Read the model definition and answer for the solid it produces. Units are mm, in the model's axes. A direction names the side the tool comes from. Give positions to 0.01 mm unless a question says otherwise; leave off trailing zeros. Loops run counter-clockwise (first coordinate to the right, second up) from the corner with the lowest first, then second, coordinate; pieces in that order, holes last. Notation, with made-up numbers: (-5.5, -26) -> (41.5, -26) arc R15 cw to (41.5, -2) -> close; hole circle Ø10 at (25, -38). An arc over 180 degrees is marked (long way). Return JSON: item names as keys, results as strings. Group by question number.
from build123d import *

# Parameters (mm, degrees)
F0_R     = 25.4
F1_DEPTH = 1.27
F3_R     = 1.27
F4_DEPTH = 76.2
F5_R     = 28.9937476924
F6_DEPTH = 38.1


# Not quite as in the source:
# - a fillet or chamfer that OpenCascade refuses, or shapes differently, is made with other operations: its cross-section is extruded or revolved along the edge and cut away or added


with BuildPart() as f1:
    # F0 (on Top) → F1 (new body)
    with BuildSketch(Plane.XY):
        Circle(F0_R)
    extrude(amount=F1_DEPTH)

    # F2: fillet of radius 5.08 on 1 edges, made by hand

    # F2_s1 → F2_t2 (revolve, cut)
    with BuildSketch(Plane.XZ):
        with BuildLine():
            ThreePointArc((25.4, 0), (23.8359470592, 0.9419048812), (22.0398958349, 1.27))
            Line((22.0398958349, 1.27), (25.4, 1.27))
            Line((25.4, 1.27), (25.4, 0))
        make_face()
    revolve(axis=Axis((0, 0, 1.27), (0, 0, 1)), mode=Mode.SUBTRACT)

    # F3 (on face) → F4 (join)
    with BuildSketch(Plane.XY.offset(1.27)):
        Circle(F3_R)
    extrude(amount=F4_DEPTH)

    # F5 (on face) → F6 (join)
    with BuildSketch(Plane.XY.offset(77.47)):
        with Locations((-1.27, 0)):
            Circle(F5_R)
    extrude(amount=F6_DEPTH)


solid = f1.part
1. Section B-B on x = 0 is taken. Determine the outline of the cut face in (y, z).
2. Flat-ended cylindrical pins translate along their axes: pin 1 Ø3 at (y, z) = (21.5, 85) entering from +X; pin 2 Ø4 at (y, z) = (-2.5, 90.5) entering from -X. Find the tip coordinate at first contact, or state that the pin passes through.
3. Straight lines are drawn through the part: line 1 (Z direction, x = -12.5, y = 18.5); line 2 (Z direction, x = -26, y = -2.5); line 3 (Z direction, x = 24, y = 0). For each, find the intervals that lie inside material, in ascending order. Write a range as from..to.
4. Which of the six approach directions +Z, -Z, +X, -X, +Y, -Y give full straight-line access (tool end or side, diameter ignored) to faces 1 (the cylindrical face through (-0.17, 1.26, 38.84)), 2 (the cylindrical face through (-7.555, -28.304, 96.253))?
5. Determine the mould class of faces 3 (the flat face through (-2, 0, 115.57)), 4 (the flat face through (0, 0, 0)), 5 (the flat face through (-2, 0, 77.47)) for opening direction Z: pulls with the +Z half, pulls with the -Z half, needs draft (parallel to the pull), parting line crosses it, or undercut.
6. Section A-A on z = 17.5 is taken. Determine the outline of the cut face in (x, y), then the cut area to 3 significant figures.
Completed:
{
 "1": {"outline": "(-28.97, 77.47) -> (-1.27, 77.47) -> (-1.27, 1.27) -> (-22.04, 1.27) arc R5.08 ccw to (-25.4, 0) -> (25.4, 0) arc R5.08 ccw to (22.04, 1.27) -> (1.27, 1.27) -> (1.27, 77.47) -> (28.97, 77.47) -> (28.97, 115.57) -> (-28.97, 115.57) -> close"},
 "2": {"pin 1": "stops at x = 19.72", "pin 2": "stops at x = -30.26"},
 "3": {"line 1": "z = 0..1.26, 77.47..115.57", "line 2": "z = 77.47..115.57", "line 3": "z = 0..0.88, 77.47..115.57"},
 "4": {"face 1": "none", "face 2": "+Z, -Z"},
 "5": {"face 3": "pulls with the +Z half", "face 4": "pulls with the -Z half", "face 5": "undercut"},
 "6": {"outline": "circle Ø2.54 at (0, 0)", "area": "5.07 mm²"}
}
